Here's how the part is built. I have some questions about the finished solid (model axes, mm). A direction names the side the tool comes from. Round coordinates to 2 decimals unless told otherwise and drop trailing zeros. Order: outer loops, then holes, each group sorted by start corner. A loop starts at its lowest first (then second) coordinate and runs counter-clockwise, first axis right, second up. Notation, with made-up numbers: (-29.75, -7.75) - (8.25, -7.75) arc R21 cw to (8.25, 8.25) - close; hole circle Ø9 at (65.25, 62). An arc over 180 degrees is marked (long way). Answer as a JSON object with one key per item and string values.
```python
from build123d import *

# Parameters (mm, degrees)
SKETCH1_R           = 19.05
BOSS_EXTRUDE1_DEPTH = 50.8


with BuildPart() as part:
    # Sketch1 → Boss-Extrude1 (new body)
    with BuildSketch(Plane.XY):
        with BuildLine():
            Line((-63.5, 0), (63.5, 0))
            Line((63.5, 0), (63.5, 63.5))
            Line((63.5, 63.5), (50.8, 63.5))
            ThreePointArc((50.8, 63.5), (0, 114.3), (-50.8, 63.5))
            Line((-50.8, 63.5), (-63.5, 63.5))
            Line((-63.5, 63.5), (-63.5, 0))
        make_face()
        with Locations((0, 63.5)):
            Circle(SKETCH1_R, mode=Mode.SUBTRACT)
    extrude(amount=BOSS_EXTRUDE1_DEPTH)


solid = part.part
```
1. If I drill on L1, parallel to Y at x = 0, z = 14.5; L2, parallel to Y at x = -56.5, z = 23; L3, parallel to Y at x = 9, z = 49, over which ranges is the centre line in solid material (lowest first)? Write a range as [from, to].
Responses:
{"L1": "[0, 44.45], [82.55, 114.3]", "L2": "[0, 63.5]", "L3": "[0, 46.71], [80.29, 113.5]"}
2. Imagine slicing it at B-B (z = 30.5). List the corners of the cut face in (x, y) for me.
Responses:
{"outline": "(-63.5, 0) - (63.5, 0) - (63.5, 63.5) - (50.8, 63.5) arc R50.8 ccw to (-50.8, 63.5) - (-63.5, 63.5) - close; hole circle Ø38.1 at (0, 63.5)"}
3. For P1, Ø12, axis at x = -28.5, z = 24.5, coming from the +Y side; P2, Ø12, axis at x = 5.5, z = 39, coming from the +Y side; P3, Ø1.5, axis at y = 96.5, z = 26.5, coming from the -X side, each with a flat end and sliding along its axis, tell me the tip position at first contact or that it passes through.
Responses:
{"P1": "y = 109.05", "P2": "y = 114.3", "P3": "x = -39.25"}
4. Imagine slicing it at A-A (x = 0). List the corners of the cut face in (y, z) for me, plus the area to 3 significant figures.
Responses:
{"outline": "(0, 0) - (44.45, 0) - (44.45, 50.8) - (0, 50.8) - close; (82.55, 0) - (114.3, 0) - (114.3, 50.8) - (82.55, 50.8) - close", "area": "3,870 mm2"}
5. Thinking about a two-plate mould opening in X: for faces 1 (the face through (-4.13, 44.903, 25.044)), 2 (the face through (-63.5, 32, 25)), 3 (the face through (1.117, 114.288, 25.044)), 4 (the face through (-1, 0, 25)), which applies, pulls with the +X half, pulls with the -X half, needs draft (parallel to the pull), parting line crosses it, or undercut?
Responses:
{"face 1": "undercut", "face 2": "pulls with the -X half", "face 3": "parting line crosses it", "face 4": "needs draft"}
6. For faces 5 (the face through (-57, 63.5, 25)), 6 (the face through (57, 63.5, 25)), 7 (the face through (13, 45, 50.8)), which set-ups out of +Z, -Z, +X, -X, +Y, -Y let a thin tool reach every point of the face, with its end or its side?
Responses:
{"face 5": "+Z, -Z, -X, +Y", "face 6": "+Z, -Z, +X, +Y", "face 7": "+Z, +X, -X, +Y, -Y"}
7. Imagine slicing it at D-D (x = -34.5). List the corners of the cut face in (y, z) for me, plus the area to 3 significant figures.
Responses:
{"outline": "(0, 0) - (100.79, 0) - (100.79, 50.8) - (0, 50.8) - close", "area": "5,120 mm2"}
8. Imagine slicing it at C-C (y = 69.5). List the corners of the cut face in (x, z) for me, plus the area to 3 significant figures.
Responses:
{"outline": "(-50.44, 0) - (-18.08, 0) - (-18.08, 50.8) - (-50.44, 50.8) - close; (18.08, 0) - (50.44, 0) - (50.44, 50.8) - (18.08, 50.8) - close", "area": "3,290 mm2"}
